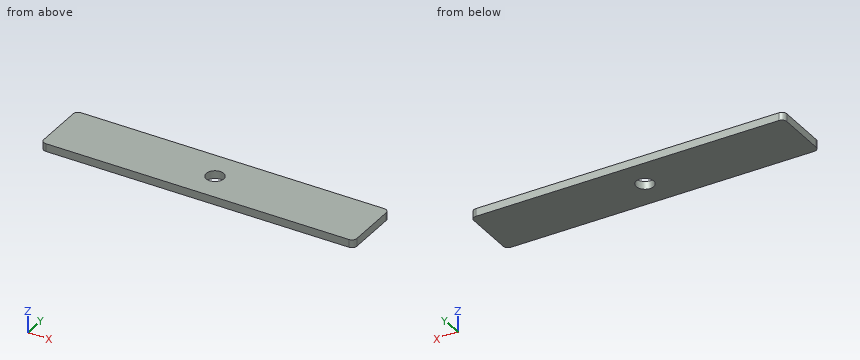
Autodesk Inventor part; units mm, degrees
ref_plane "YZ Plane" through (0, 0, 0) normal (1, 0, 0) x (0, 1, 0)
ref_plane "XZ Plane" through (0, 0, 0) normal (0, 1, 0) x (-1, 0, 0)
ref_plane "XY Plane" through (0, 0, 0) normal (0, 0, 1) x (1, 0, 0)
sketch "Sketch1" plane through (0, 0, 0) normal (0, 0, 1) x (1, 0, 0)
  line L0 (-101.6, -19.05) -> (101.6, -19.05)
  line L1 (101.6, -19.05) -> (101.6, 19.05)
  line L2 (101.6, 19.05) -> (-101.6, 19.05)
  line L3 (-101.6, 19.05) -> (-101.6, -19.05)
  line L4 (-101.6, -19.05) -> (101.6, 19.05) construction
  line L5 (101.6, -19.05) -> (-101.6, 19.05) construction
  circle A0 centre (0, 0) radius 5.715
  dimension "d0" = 203.2
  dimension "d1" = 38.1
  dimension "d2" = 11.43
extrude "Extrusion1" add sketch "Sketch1" along normal blind 5.08
fillet "Fillet1" radius 3.175 4 edges at (-101.6, 19.05, 2.54) (-101.6, -19.05, 2.54) (101.6, 19.05, 2.54) (101.6, -19.05, 2.54)
properties part number "Stress Tester Sample"
Part model, mm, in its own coordinate system. Round coordinates to 2 decimals unless told otherwise and drop trailing zeros. Loops run counter-clockwise (first coordinate to the right, second up) from the corner with the lowest first, then second, coordinate; pieces in that order, holes last. Notation, with made-up numbers: (47.25, -6.5) - (105.25, -6.5) arc R26 ccw to (105.25, 14.5) - close; hole circle Ø11 at (-26.5, -15). An arc over 180 degrees is marked (long way). Answer as a JSON object with one key per item and string values.
Item 1: Band-saw the part on B-B on x = 0. List the corners of the cut face in (y, z) (3 decimals).
Output:
{"outline": "(-19.05, 0) - (-5.715, 0) - (-5.715, 5.08) - (-19.05, 5.08) - close; (5.715, 0) - (19.05, 0) - (19.05, 5.08) - (5.715, 5.08) - close"}
Item 2: Wall check: L1, parallel to Y at x = 0, z = 3.45 (3 decimals); L2, parallel to X at y = -3, z = 2.7; L3, parallel to X at y = -4.5, z = 2.75. Give the ranges that are in metal, low to high.
Output:
{"L1": "-19.05 to -5.715, 5.715 to 19.05", "L2": "-101.6 to -4.86, 4.86 to 101.6", "L3": "-101.6 to -3.52, 3.52 to 101.6"}
Item 3: Band-saw the part on A-A on y = 0. List the corners of the cut face in (x, z) (3 decimals).
Output:
{"outline": "(-101.6, 0) - (-5.715, 0) - (-5.715, 5.08) - (-101.6, 5.08) - close; (5.715, 0) - (101.6, 0) - (101.6, 5.08) - (5.715, 5.08) - close"}
